```python
from build123d import *

# Parameters (mm, degrees)
CYLINDER004_R             = 7.5
CYLINDER004_DEPTH         = 240
CYLINDER005_R             = 7.5
CYLINDER005_DEPTH         = 240
BOX030_W                  = 45
BOX030_H                  = 60
BOX030_DEPTH              = 100
BOX031_W                  = 45
BOX031_H                  = 60
BOX031_DEPTH              = 100
BOX032_W                  = 120
BOX032_H                  = 30
BOX032_DEPTH              = 120
BOX028_W                  = 170
BOX028_H                  = 15
BOX028_DEPTH              = 180
BOX033_W                  = 25
BOX033_H                  = 25
BOX033_DEPTH              = 100
CYLINDER006_R             = 30
CYLINDER006_DEPTH         = 80
CYLINDER007_R             = 25
CYLINDER007_DEPTH         = 80
BOX029_W                  = 215
BOX029_H                  = 25
BOX029_DEPTH              = 50
FUSION005_PLACEMENT_ANGLE = 180


with BuildPart() as cylinder004:
    # Cylinder004 → Cylinder004 (new body)
    with BuildSketch(Plane(origin=(-12.5, 33.5, -55), x_dir=(1, 0, 0), z_dir=(0, 0, 1))):
        Circle(CYLINDER004_R)
    extrude(amount=CYLINDER004_DEPTH)


with BuildPart() as cylinder005:
    # Cylinder005 → Cylinder005 (new body)
    with BuildSketch(Plane(origin=(182.5, 33.5, -55), x_dir=(1, 0, 0), z_dir=(0, 0, 1))):
        Circle(CYLINDER005_R)
    extrude(amount=CYLINDER005_DEPTH)


with BuildPart() as cube025:
    # Box030 → Box030 (new body)
    with BuildSketch(Plane(origin=(-45, -1, 25), x_dir=(1, 0, 0), z_dir=(0, 0, 1))):
        with Locations((22.5, 30)):
            Rectangle(BOX030_W, BOX030_H)
    extrude(amount=BOX030_DEPTH)


with BuildPart() as cube026:
    # Box031 → Box031 (new body)
    with BuildSketch(Plane(origin=(170, -1, 25), x_dir=(1, 0, 0), z_dir=(0, 0, 1))):
        with Locations((22.5, 30)):
            Rectangle(BOX031_W, BOX031_H)
    extrude(amount=BOX031_DEPTH)


with BuildPart() as cube027:
    # Box032 → Box032 (new body)
    with BuildSketch(Plane(origin=(25, -1, 25), x_dir=(1, 0, 0), z_dir=(0, 0, 1))):
        with Locations((60, 15)):
            Rectangle(BOX032_W, BOX032_H)
    extrude(amount=BOX032_DEPTH)


with BuildPart() as cut008:
    # Box028 → Box028 (new body)
    with BuildSketch(Plane.XY):
        with Locations((85, 7.5)):
            Rectangle(BOX028_W, BOX028_H)
    extrude(amount=BOX028_DEPTH)

    # Cut008: cut Cube027
    add(cube027.part, mode=Mode.SUBTRACT)


with BuildPart() as cube028:
    # Box033 → Box033 (new body)
    with BuildSketch(Plane(origin=(72.5, 76.5, -155), x_dir=(1, 0, 0), z_dir=(0, -1, 0))):
        with Locations((12.5, 12.5)):
            Rectangle(BOX033_W, BOX033_H)
    extrude(amount=BOX033_DEPTH)


with BuildPart() as cylinder006:
    # Cylinder006 → Cylinder006 (new body)
    with BuildSketch(Plane(origin=(85, 34, -180), x_dir=(1, 0, 0), z_dir=(0, 0, 1))):
        Circle(CYLINDER006_R)
    extrude(amount=CYLINDER006_DEPTH)


with BuildPart() as cut009:
    # Cylinder007 → Cylinder007 (new body)
    with BuildSketch(Plane(origin=(45, 33.5, -165), x_dir=(0, 0, -1), z_dir=(1, 0, 0))):
        Circle(CYLINDER007_R)
    extrude(amount=CYLINDER007_DEPTH)

    # Fusion004: union Cylinder006
    add(cylinder006.part)

    # Cut009: cut Cube028
    add(cube028.part, mode=Mode.SUBTRACT)


with BuildPart() as standard001:
    # Box029 → Box029 (new body)
    with BuildSketch(Plane(origin=(-22.5, 21, -100), x_dir=(1, 0, 0), z_dir=(0, 0, 1))):
        with Locations((107.5, 12.5)):
            Rectangle(BOX029_W, BOX029_H)
    extrude(amount=BOX029_DEPTH)

    # Fusion005: union Cylinder004, Cylinder005, Cube025, Cube026, Cut008, Cut009
    add(cylinder004.part)
    add(cylinder005.part)
    add(cube025.part)
    add(cube026.part)
    add(cut008.part)
    add(cut009.part)


with BuildPart() as standard001_1:
    # Fusion005 placement: moved
    add(standard001.part.moved(Location((170, 407, 0))).rotate(Axis((170, 407, 0), (0, 0, 1)), FUSION005_PLACEMENT_ANGLE))


solid = standard001_1.part
```
Input: part model. Units: mm. Frame: model coordinates. A direction names the side the tool comes from. Give positions to 0.01 mm unless a question says otherwise; leave off trailing zeros. Order: outer loops, then holes, each group sorted by start corner. A loop starts at its lowest first (then second) coordinate and runs counter-clockwise, first axis right, second up. Notation, with made-up numbers: M 72.25,5 L 123.25,5 A20 ccw 123.25,9 Z; hole C 75.25,52 d10. An arc over 180 degrees is marked long. One line per question, with ' | ' between items. Start each with the question number.
1. Section query C-C (z = 153). Return the cut outline in (x, y).
2. Section query B-B (z = 33). Return the cut outline in (x, y).
3. First-contact query: pin 1 Ø6 at (y, z) = (378, -43) entering from -X; pin 2 Ø7.5 at (y, z) = (372, -86) entering from +X; pin 3 Ø15 at (y, z) = (361.5, -174) entering from -X. Flat tips, straight axial feed; report the tip coordinate or a pass-through.
4. Material intervals for probe 1 along X at (y, z) = (402, 132); probe 2 along Z at (x, y) = (107, 399); probe 3 along Z at (x, y) = (115, 374.5), sorted ascending. Write a range as [from, to].
5. Section query A-A (x = 85). Return the cut outline in (y, z), and give its area (3 significant figures).
6. Pull-direction query (Z, two-part tool) for faces 1 (the face through (175.57, 376.37, -13.02)), 2 (the face through (183, 373, 185)), 3 (the face through (170, 400, 152)); classes: released by +Z, released by -Z, zero draft, split by the parting line, or undercut.
7. Access query for faces 4 (the face through (45, 373, -165)), 5 (the face through (170, 370, 74)), 6 (the face through (97.5, 373, -143)), 7 (the face through (85, 392, -100)), 8 (the face through (175.57, 376.37, 154.58)). Directions: +Z, -Z, +X, -X, +Y, -Y. A direction counts if a zero-diameter tool reaches every point of the face in a straight line with its end or side. Return the directions, or none.
8. Section query D-D (x = -12.5). Return the cut outline in (y, z).
Here are the results:
1) outline: C -12.5,373.5 d15; M 0,392 L 170,392 L 170,407 L 0,407 Z; C 182.5,373.5 d15
2) outline: M -45,348 L 0,348 L 0,392 L 25,392 L 25,407 L 0,407 L 0,408 L -45,408 Z; M 145,392 L 170,392 L 170,348 L 215,348 L 215,408 L 170,408 L 170,407 L 145,407 Z
3) pin 1: x = -19.85 | pin 2: x = 192.5 | pin 3: x = 45
4) probe 1: [0, 25], [145, 170] | probe 2: [0, 25], [145, 180] | probe 3: [-189.98, -140.02], [-100, -50]
5) outline: M 343,-180 L 353.5,-180 A25 ccw 393.5,-180 L 403,-180 L 403,-155 L 343,-155 Z; M 343,-130 L 403,-130 L 403,-100 L 386,-100 L 386,-50 L 361,-50 L 361,-100 L 343,-100 Z; M 392,0 L 407,0 L 407,25 L 392,25 Z; M 392,145 L 407,145 L 407,180 L 392,180 Z | area: 5,730 mm²
6) face 1: undercut | face 2: released by +Z | face 3: zero draft
7) face 4: -Z, -X, +Y, -Y | face 5: +Z, -Y | face 6: +Y, -Y | face 7: +X, -X, +Y | face 8: +Z
8) outline: M 348,25 L 366,25 L 366,-50 L 361,-50 L 361,-100 L 386,-100 L 386,-50 L 381,-50 L 381,25 L 408,25 L 408,125 L 381,125 L 381,185 L 366,185 L 366,125 L 348,125 Z
